Read the model definition and answer for the solid it produces. Units are mm, in the model's axes. Face numbers are marked on the shaded views. A direction names the side the tool comes from. Round coordinates to 2 decimals unless told otherwise and drop trailing zeros. Order: outer loops, then holes, each group sorted by start corner. A loop starts at its lowest first (then second) coordinate and runs counter-clockwise, first axis right, second up. Notation, with made-up numbers: (8, 64.25) - (39, 64.25) arc R17 ccw to (39, 71.25) - close; hole circle Ø9 at (78.25, -6.75). An arc over 180 degrees is marked (long way). One line per question, with ' | ' between items. Start each with the question number.
1) For the marked faces 1 and 2, determine the directions among +Z, -Z, +X, -X, +Y, -Y from which every point of the face is accessible in a straight line to the end or side of a thin tool.
2) Straight lines are drawn through the part: line 1 (Y direction, x = 130, z = 0); line 2 (X direction, y = -9.5, z = 23.5); line 3 (Z direction, x = 99, y = 3). For each, find the intervals that lie inside material, in ascending order. Write a range as from..to.
3) The part is cut by section D-D, the plane z = -16. Give the vertices of the cut face in (x, y).
4) The part is cut by section B-B, the plane y = 20. Give the vertices of the cut face in (x, z).
5) Flat-ended cylindrical pins translate along their axes: pin 1 (1 mm diameter, centred on y = 21.5, z = 22, fed in from +X); pin 2 (1 mm diameter, centred on x = 64, y = -11.5, fed in from -Z); pin 3 (1.5 mm diameter, centred on x = 92, y = -15.5, fed in from +Z); pin 4 (10 mm diameter, centred on x = 90.5, y = 17.5, fed in from -Z). Find the tip coordinate at first contact, or state that the pin passes through.
6) The part is cut by section C-C, the plane x = 95.5. Give the vertices of the cut face in (y, z).
7) The part is cut by section A-A, the plane z = 0. Give the vertices of the cut face in (x, y) (3 decimals), plus the area to 3 significant figures.
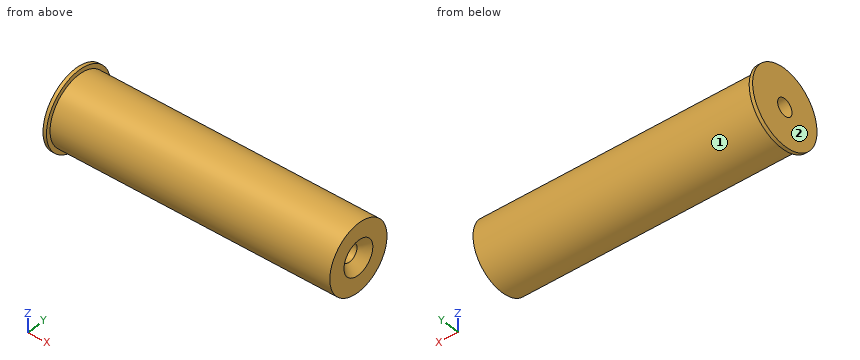
from build123d import *

# Parameters (mm, degrees)
SKETCH1_R           = 25.2
BOSS_EXTRUDE1_DEPTH = 208.28
SKETCH2_R           = 28.375
BOSS_EXTRUDE2_DEPTH = 2.54
SKETCH4_R           = 6.35
CUT_EXTRUDE1_DEPTH  = 213.110442105
CHAMFER1_SIZE       = 6.35


with BuildPart() as part:
    # Sketch1 → Boss-Extrude1 (new body)
    with BuildSketch(Plane(origin=(0, 0, 0), x_dir=(0, 0, -1), z_dir=(1, 0, 0))):
        Circle(SKETCH1_R)
    extrude(amount=BOSS_EXTRUDE1_DEPTH)

    # Sketch2 → Boss-Extrude2 (add)
    with BuildSketch(Plane.ZY):
        Circle(SKETCH2_R)
    extrude(amount=-BOSS_EXTRUDE2_DEPTH)

    # Sketch4 → Cut-Extrude1 (cut, through all)
    with BuildSketch(Plane(origin=(208.28, 0, 0), x_dir=(0, 0, -1), z_dir=(1, 0, 0))):
        Circle(SKETCH4_R)
    extrude(amount=-CUT_EXTRUDE1_DEPTH, mode=Mode.SUBTRACT)

    # Chamfer1
    chamfer1_edges = [part.edges().sort_by_distance(p)[0] for p in [
        (208.28, 0, 6.35),
    ]]
    chamfer(chamfer1_edges, length=CHAMFER1_SIZE)


solid = part.part
Values:
1) face 1: +X | face 2: +Z, -Z, -X, +Y, -Y
2) line 1: y = -25.2..-6.35, 6.35..25.2 | line 2: x = 0..2.54 | line 3: z = -25.02..-5.6, 5.6..25.02
3) outline: (0, -23.43) - (2.54, -23.43) - (2.54, -19.47) - (208.28, -19.47) - (208.28, 19.47) - (2.54, 19.47) - (2.54, 23.43) - (0, 23.43) - close
4) outline: (0, -20.13) - (2.54, -20.13) - (2.54, -15.33) - (208.28, -15.33) - (208.28, 15.33) - (2.54, 15.33) - (2.54, 20.13) - (0, 20.13) - close
5) pin 1: passes through | pin 2: stops at z = -22.67 | pin 3: stops at z = 20.43 | pin 4: stops at z = -21.88
6) outline: circle Ø50.4 at (0, 0); hole circle Ø12.7 at (0, 0)
7) outline: (0, -28.375) - (2.54, -28.375) - (2.54, -25.2) - (208.28, -25.2) - (208.28, -12.7) - (201.93, -6.35) - (0, -6.35) - close; (0, 6.35) - (201.93, 6.35) - (208.28, 12.7) - (208.28, 25.2) - (2.54, 25.2) - (2.54, 28.375) - (0, 28.375) - close | area: 7,830 mm^2
